Autodesk Fusion 360 part; units mm, degrees
sketch "Esquisse1" plane through (0, 0, 0) normal (0, 0, 1) x (1, 0, 0)
  line L0 (0, 0) -> (45, 0)
  line L1 (45, 0) -> (45, 22)
  line L2 (45, 22) -> (0, 22)
  line L3 (0, 22) -> (0, 0)
  dimension "d1" = 45
  dimension "d2" = 22
extrude "Extrusion1" add sketch "Esquisse1" along normal blind 2
sketch "Esquisse2" plane through (0, 0, 0) normal (0, 0, -1) x (1, 0, 0)
  line L0 (0, 0) -> (0, -22)
  line L1 (0, -22) -> (45, -22)
  line L2 (45, -22) -> (45, 0)
  line L3 (45, 0) -> (0, 0)
  line L4 (1.4, -20.6) -> (43.6, -20.6)
  line L5 (43.6, -20.6) -> (43.6, -1.4)
  line L6 (43.6, -1.4) -> (1.4, -1.4)
  line L7 (1.4, -1.4) -> (1.4, -20.6)
  dimension "d5" = -1.4
extrude "Extrusion2" add sketch "Esquisse2" along normal blind 1.7 contours L4 L5 L6 L7
fillet "Congé1" radius 1.5 4 edges at (0, 0, 1) (45, 0, 1) (45, 22, 1) (0, 22, 1)
chamfer "Chanfrein1" distance 0.3 angle 45 4 edges at (22.5, 20.6, -1.7) (1.4, 11, -1.7) (22.5, 1.4, -1.7) (43.6, 11, -1.7)
fillet "Congé2" radius 0.5 8 edges at (0.4393, 21.5607, 2) (0, 11, 2) (0.4393, 0.4393, 2) (22.5, 0, 2) (44.5607, 0.4393, 2) (45, 11, 2) (44.5607, 21.5607, 2) (22.5, 22, 2)
hole "Perçage1" at (15.166, 10.5, 2) direction (0, 0, -1) diameter 1.5 depth 9 tip angle 180 counterbore diameter 3 counterbore depth 2
pattern_linear "Réseau R1" count 2 spacing 14.666 along (1, 0, 0) of "Perçage1"
Read the model definition and answer for the solid it produces. Units are mm, in the model's axes. A direction names the side the tool comes from. Round coordinates to 2 decimals unless told otherwise and drop trailing zeros. Order: outer loops, then holes, each group sorted by start corner. A loop starts at its lowest first (then second) coordinate and runs counter-clockwise, first axis right, second up.
1) For faces 4 (the face through (29, 10, 0)), 5 (the face through (22, 20.6, -1)), 6 (the face through (1.4, 11, -1)), determine the directions among +Z, -Z, +X, -X, +Y, -Y from which every point of the face is accessible in a straight line to the end or side of a thin tool.
2) The part is cut by section D-D on y = 19.75. Write down the section's boundary in (x, z).
3) The part is cut by section C-C on z = 0.8. Write down the section's boundary in (x, y), plus the area to 3 significant figures.
4) Flat-ended cylindrical pins translate along their axes: pin 1 (2.5 mm diameter, centred on x = 15, y = 11, fed in from +Z); pin 2 (2.5 mm diameter, centred on x = 15.166, y = 10.5, fed in from +Z); pin 3 (0.7 mm diameter, centred on y = 10.5, z = -0.5, fed in from +X); pin 4 (0.7 mm diameter, centred on y = 14.5, z = -0.5, fed in from -X). Find the tip coordinate at first contact, or state that the pin passes through.
5) The mould has two halves that part along Y. Classify faces 1 (the face through (23, 22, 1)), 2 (the face through (45, 11, 1)), 3 (the face through (14, 10, 0)): released by +Y, released by -Y, zero draft, split by the parting line, or undercut.
6) The part is cut by section A-A on y = 10.5. Write down the section's boundary in (x, z).
7) The part is cut by section B-B on x = 27. Write down the section's boundary in (y, z).
8) Straight lines are drawn through the part: L1, parallel to X at y = 10.5, z = -1.2; L2, parallel to Y at x = 31.5, z = -0.9; L3, parallel to X at y = 10.25, z = 1.65. For each, find the intervals that lie inside material, in ascending order.
Resolved:
1. face 4: +Z
1. face 5: -Z, +X, -X, +Y
1. face 6: -Z, -X, +Y, -Y
2. outline: (0, 0) - (1.4, 0) - (1.4, -1.4) - (1.7, -1.7) - (43.3, -1.7) - (43.6, -1.4) - (43.6, 0) - (45, 0) - (45, 1.5) arc R0.5 ccw to (44.5, 2) - (0.5, 2) arc R0.5 ccw to (0, 1.5) - close
3. outline: (0, 1.5) arc R1.5 ccw to (1.5, 0) - (43.5, 0) arc R1.5 ccw to (45, 1.5) - (45, 20.5) arc R1.5 ccw to (43.5, 22) - (1.5, 22) arc R1.5 ccw to (0, 20.5) - close; hole circle Ø3 at (15.17, 10.5); hole circle Ø3 at (29.83, 10.5)
3. area: 974 mm2
4. pin 1: stops at z = 2
4. pin 2: stops at z = 0
4. pin 3: stops at x = 43.6
4. pin 4: stops at x = 1.4
5. face 1: released by +Y
5. face 2: zero draft
5. face 3: undercut
6. outline: (0, 0) - (1.4, 0) - (1.4, -1.4) - (1.7, -1.7) - (14.42, -1.7) - (14.42, 0) - (13.67, 0) - (13.67, 2) - (0.5, 2) arc R0.5 ccw to (0, 1.5) - close; (15.92, -1.7) - (29.08, -1.7) - (29.08, 0) - (28.33, 0) - (28.33, 2) - (16.67, 2) - (16.67, 0) - (15.92, 0) - close; (30.58, -1.7) - (43.3, -1.7) - (43.6, -1.4) - (43.6, 0) - (45, 0) - (45, 1.5) arc R0.5 ccw to (44.5, 2) - (31.33, 2) - (31.33, 0) - (30.58, 0) - close
7. outline: (0, 0) - (1.4, 0) - (1.4, -1.4) - (1.7, -1.7) - (20.3, -1.7) - (20.6, -1.4) - (20.6, 0) - (22, 0) - (22, 1.5) arc R0.5 ccw to (21.5, 2) - (0.5, 2) arc R0.5 ccw to (0, 1.5) - close
8. L1: x = 1.4 to 14.42, 15.92 to 29.08, 30.58 to 43.6
8. L2: y = 1.4 to 20.6
8. L3: x = 0.02 to 13.69, 16.65 to 28.35, 31.31 to 44.98
